Part model, mm, in its own coordinate system. A direction names the side the tool comes from. Coordinates: 2 decimals unless noted, no trailing zeros. Loops run counter-clockwise (first coordinate to the right, second up) from the corner with the lowest first, then second, coordinate; pieces in that order, holes last. Notation, with made-up numbers: (25, 0) -> (82, 0) arc R15 ccw to (82, 11) -> close; hole circle Ø6 at (-6, -39). An arc over 180 degrees is marked (long way). Use one line per item in the form item = value. Start each with the question number.
(1) Mould opens along X. For faces 3 (the flat face through (20, 10, 0)), 4 (the flat face through (5, 30, 0)), 5 (the flat face through (-25, 25, 5)) say: +X half, -X half, draft (parallel to the pull), parting line (faces both ways), or undercut.
(2) Band-saw the part on B-B on y = 14. Give the cut face in (x, z), then the cut area to 3 significant figures.
(3) Band-saw the part on C-C on z = -17. Give the cut face in (x, y), then the cut area to 3 significant figures.
(4) Band-saw the part on A-A on z = 10. Give the cut face in (x, y).
(5) Band-saw the part on D-D on y = 7.5. Give the cut face in (x, z), then the cut area to 3 significant figures.
(6) Drill centre lines: L1, parallel to X at y = 4, z = 3; L2, parallel to X at y = 29.5, z = 2; L3, parallel to Y at x = 7.5, z = 16. Where is each one in solid material? Low to high. Write a range as [from, to].
(7) 3-axis set-ups, long thin cutter, end or side, ignore diameter. For faces 1 (the flat face through (-5, 25, 5)), 2 (the flat face through (35, 5, 0)): which of +Z, -Z, +X, -X, +Y, -Y reach the whole face in a straight line?
(8) Pin check, flat tips, straight feed: P1, Ø15, axis at y = 22.5, z = 12, coming from the +X side; P2, Ø6, axis at x = -19, y = 29, coming from the +Z side. Stop position of each tip, or through.
```python
from build123d import *

# Parameters (mm, degrees)
SKETCH1_W           = 70
SKETCH1_H           = 40
BOSS_EXTRUDE1_DEPTH = 10
SKETCH2_W           = 40
SKETCH2_H           = 40
BOSS_EXTRUDE2_DEPTH = 40
SKETCH3_W           = 20
SKETCH3_H           = 30
CUT_EXTRUDE1_DEPTH  = 65.226162893


with BuildPart() as part:
    # Sketch1 → Boss-Extrude1 (new body)
    with BuildSketch(Plane(origin=(0, 0, 0), x_dir=(1, 0, 0), z_dir=(0, 1, 0))):
        Rectangle(SKETCH1_W, SKETCH1_H)
    extrude(amount=BOSS_EXTRUDE1_DEPTH)

    # Sketch2 → Boss-Extrude2 (add)
    with BuildSketch(Plane(origin=(0, 10, 0), x_dir=(1, 0, 0), z_dir=(0, 1, 0))):
        with Locations((-15, 0)):
            Rectangle(SKETCH2_W, SKETCH2_H)
    extrude(amount=BOSS_EXTRUDE2_DEPTH)

    # Sketch3 → Cut-Extrude1 (cut, through all)
    with BuildSketch(Plane(origin=(0, 50, 0), x_dir=(1, 0, 0), z_dir=(0, 1, 0))):
        with Locations((-15, -5)):
            Rectangle(SKETCH3_W, SKETCH3_H)
    extrude(amount=-CUT_EXTRUDE1_DEPTH, mode=Mode.SUBTRACT)


solid = part.part
```
A:
q1.face_3 = draft
q1.face_4 = +X half
q1.face_5 = undercut
q2.outline = (-35, -20) -> (5, -20) -> (5, 20) -> (-5, 20) -> (-5, -10) -> (-25, -10) -> (-25, 20) -> (-35, 20) -> close
q2.area = 1,000 mm²
q3.outline = (-35, 0) -> (35, 0) -> (35, 10) -> (5, 10) -> (5, 50) -> (-35, 50) -> close
q3.area = 2,300 mm²
q4.outline = (-35, 0) -> (-25, 0) -> (-25, 50) -> (-35, 50) -> close; (-5, 0) -> (35, 0) -> (35, 10) -> (5, 10) -> (5, 50) -> (-5, 50) -> close
q5.outline = (-35, -20) -> (35, -20) -> (35, 20) -> (-5, 20) -> (-5, -10) -> (-25, -10) -> (-25, 20) -> (-35, 20) -> close
q5.area = 2,200 mm²
q6.L1 = [-35, -25], [-5, 35]
q6.L2 = [-35, -25], [-5, 5]
q6.L3 = [0, 10]
q7.face_1 = +Z, +Y, -Y
q7.face_2 = +Z, -Z, +X, +Y, -Y
q8.P1 = 5
q8.P2 = -10
